Answer from the drawing. Dimensions are ordinates in mm from the lowest x, y and z of the part. Give positions to 0.01 mm unless a question says otherwise; leave off trailing zeros. Order: outer loops, then holes, each group sorted by start corner. A loop starts at its lowest first (then second) coordinate and runs counter-clockwise, first axis right, second up. Notation, with made-up numbers: (-24, 71.5) - (16, 71.5) arc R33 ccw to (16, 101.5) - close; hole circle Ø3 at (34.25, 62). An arc over 180 degrees is marked (long way). Write each question's results on one line, items separated by ' | '.
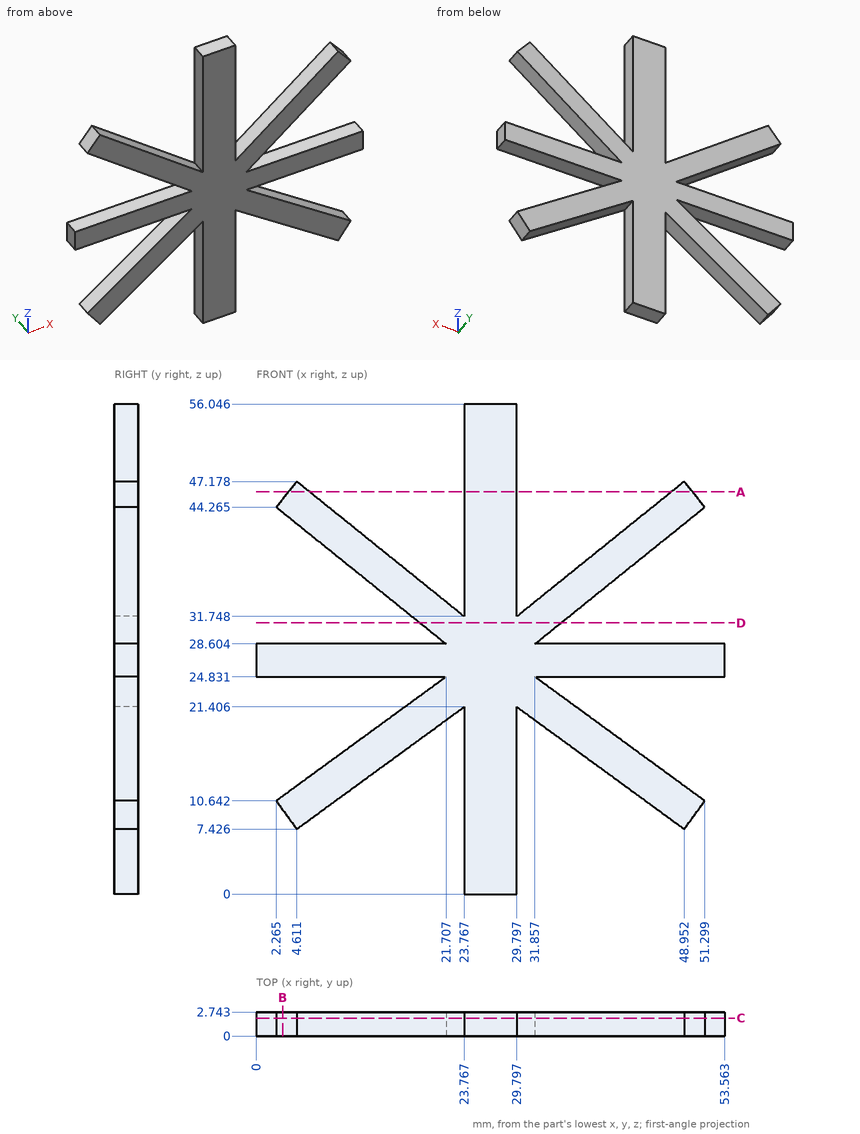
1. A cutting plane is placed at B-B, the plane x = 3. Write down the section's boundary in (y, z) (1 decimal).
Answer list:
outline: (0, 9.6) - (2.7, 9.6) - (2.7, 11.2) - (0, 11.2) - close; (0, 24.8) - (2.7, 24.8) - (2.7, 28.6) - (0, 28.6) - close; (0, 43.7) - (2.7, 43.7) - (2.7, 45.2) - (0, 45.2) - close
2. Given P1, Ø1.4, axis at y = 1.5, z = 45, coming from the +X side; P2, Ø1, axis at y = 0.5, z = 20.5, coming from the -X side; P3, Ø4, axis at x = 8, z = 21, coming from the -Y side; P4, Ø0.8, axis at y = 2, z = 12.5, coming from the -X side (1 decimal), each flat-ended and moving along its own axis, determine where each tip first touches the part or whether it passes through.
Answer list:
P1: x = 51.27 | P2: x = 15.09 | P3: through | P4: x = 4.3
3. A cutting plane is placed at A-A, the plane z = 46. Write down the section's boundary in (x, y) (1 decimal).
Answer list:
outline: (3.7, 0) - (6.1, 0) - (6.1, 2.7) - (3.7, 2.7) - close; (23.8, 0) - (29.8, 0) - (29.8, 2.7) - (23.8, 2.7) - close; (47.5, 0) - (49.9, 0) - (49.9, 2.7) - (47.5, 2.7) - close
4. A cutting plane is placed at D-D, the plane z = 31. Write down the section's boundary in (x, y).
Answer list:
outline: (18.73, 0) - (34.83, 0) - (34.83, 2.74) - (18.73, 2.74) - close
5. A cutting plane is placed at C-C, the plane y = 2.05. Write down the section's boundary in (x, z) (1 decimal).
Answer list:
outline: (0, 24.8) - (21.7, 24.8) - (2.3, 10.6) - (4.6, 7.4) - (23.8, 21.4) - (23.8, 0) - (29.8, 0) - (29.8, 21.4) - (49, 7.4) - (51.3, 10.6) - (31.9, 24.8) - (53.6, 24.8) - (53.6, 28.6) - (31.9, 28.6) - (51.3, 44.3) - (49, 47.2) - (29.8, 31.7) - (29.8, 56) - (23.8, 56) - (23.8, 31.7) - (4.6, 47.2) - (2.3, 44.3) - (21.7, 28.6) - (0, 28.6) - close
6. Straight lines are drawn through the part: line 1 (X direction, y = 0.2, z = 45.5) (1 decimal); line 2 (Z direction, x = 40.5, y = 2) (1 decimal); line 3 (Z direction, x = 19.5, y = 1.95) (1 decimal). For each, find the intervals that lie inside material, in ascending order. Write a range as [from, to].
Answer list:
line 1: [3.3, 6.7], [23.8, 29.8], [46.9, 50.3] | line 2: [13.6, 18.5], [24.8, 28.6], [35.6, 40.4] | line 3: [18.3, 23.2], [24.8, 28.6], [30.4, 35.2]
